For this review, use the dimensioned drawing (mm, ordinates from the lowest corner) and the shaded views. A direction names the side the tool comes from. Round coordinates to 2 decimals unless told otherwise and drop trailing zeros. Order: outer loops, then holes, each group sorted by start corner. A loop starts at its lowest first (then second) coordinate and runs counter-clockwise, first axis right, second up. Notation, with made-up numbers: M 0.5,84.5 L 33.5,84.5 A18 ccw 33.5,90.5 Z; hole C 58.25,8.25 d1. An arc over 180 degrees is marked long. Put each result on its own line as item: value.
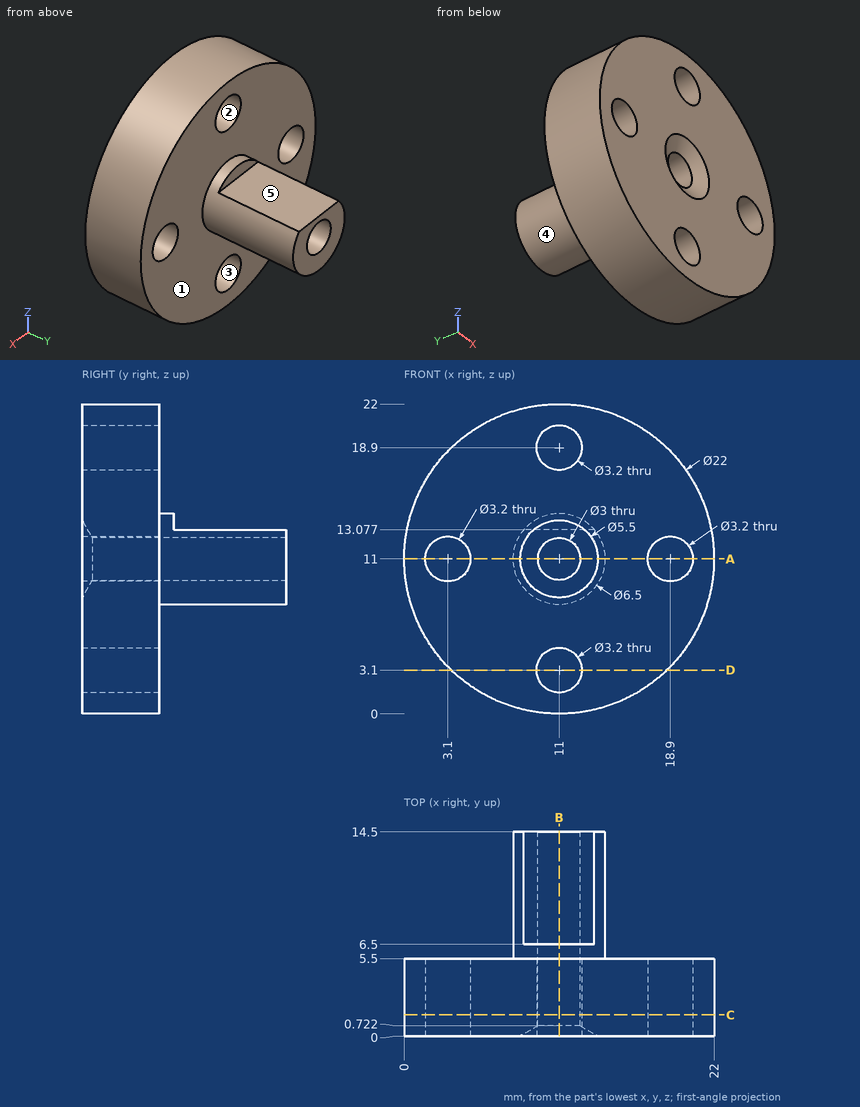
(1) Add section C-C on y = 1.5. Give the boundary of the cut face in (x, z), then the cut area to 3 significant figures.
A:
outline: C 11,11 d22; hole C 3.1,11 d3.2; hole C 11,3.1 d3.2; hole C 11,18.9 d3.2; hole C 11,11 d3; hole C 18.9,11 d3.2
area: 341 mm2
(2) To check wall thickness, follow L1, parallel to X at y = 0.75, z = 11; L2, parallel to Y at x = 9.25, z = 17.25; L3, parallel to Y at x = 13, z = 13.25. State the ranges of each line that lie inside material, in increasing order.
A:
L1: x = 0 to 1.5, 4.7 to 9.5, 12.5 to 17.3, 20.5 to 22
L2: y = 0 to 5.5
L3: y = 0 to 6.5
(3) Add section B-B on x = 11. Give the boundary of the cut face in (y, z).
A:
outline: M 0,0 L 5.5,0 L 5.5,1.5 L 0,1.5 Z; M 0,4.7 L 5.5,4.7 L 5.5,7.75 L 14.5,7.75 L 14.5,9.5 L 0.72,9.5 L 0,8.25 Z; M 0,13.75 L 0.72,12.5 L 14.5,12.5 L 14.5,13.08 L 6.5,13.08 L 6.5,14.25 L 5.5,14.25 L 5.5,17.3 L 0,17.3 Z; M 0,20.5 L 5.5,20.5 L 5.5,22 L 0,22 Z
(4) For the marked faces 1 and 2, list the 3-axis set-ups (+Z, -Z, +X, -X, +Y, -Y) from which the entire face can be reached by the end or side of a thin tool; tool diameter is ignored.
A:
face 1: +Y
face 2: +Y, -Y
(5) Add section A-A on z = 11. Give the boundary of the cut face in (x, y).
A:
outline: M 0,0 L 1.5,0 L 1.5,5.5 L 0,5.5 Z; M 4.7,0 L 8.25,0 L 9.5,0.72 L 9.5,14.5 L 7.75,14.5 L 7.75,5.5 L 4.7,5.5 Z; M 12.5,0.72 L 13.75,0 L 17.3,0 L 17.3,5.5 L 14.25,5.5 L 14.25,14.5 L 12.5,14.5 Z; M 20.5,0 L 22,0 L 22,5.5 L 20.5,5.5 Z
(6) Insertion check: pin 1 Ø8 at (x, y) = (5, 3) entering from +Z; pin 2 Ø11 at (x, z) = (15.5, 11.5) entering from +Y; pin 3 Ø1 at (x, y) = (4, 2) entering from -Z (1 decimal); pin 4 Ø4 at (x, z) = (11, 3.1) entering from +Y. Each pin has a flat end and moves straight along its axis. Give the tip position at first contact, or say it passes through.
A:
pin 1: stops at z = 21.82
pin 2: stops at y = 14.5
pin 3: stops at z = 2.1
pin 4: stops at y = 5.5
(7) Draft analysis for pull direction X (two halves, no side actions). For the marked faces 3, 4 and 5, state which applies: released by +X, released by -X, zero draft, split by the parting line, or undercut.
A:
face 3: undercut
face 4: split by the parting line
face 5: zero draft
(8) Add section D-D on z = 3.1. Give the boundary of the cut face in (x, y) (1 decimal), then the cut area to 3 significant figures.
A:
outline: M 3.3,0 L 9.4,0 L 9.4,5.5 L 3.3,5.5 Z; M 12.6,0 L 18.7,0 L 18.7,5.5 L 12.6,5.5 Z
area: 66.6 mm2
